Autodesk Inventor part; units mm, degrees
ref_plane "YZ Plane" through (0, 0, 0) normal (1, 0, 0) x (0, 1, 0)
ref_plane "XZ Plane" through (0, 0, 0) normal (0, 1, 0) x (-1, 0, 0)
ref_plane "XY Plane" through (0, 0, 0) normal (0, 0, 1) x (1, 0, 0)
sketch "Skizze1" plane through (0, 0, 0) normal (0, 0, 1) x (1, 0, 0)
  line L0 (0, 0) -> (662.5, 0)
  line L1 (662.5, 0) -> (662.5, 822.5)
  line L2 (662.5, 822.5) -> (0, 822.5)
  line L3 (0, 822.5) -> (0, 0)
  line L4 (0, 822.5) -> (40, 822.5)
  line L5 (40, 822.5) -> (40, 814.5)
  line L6 (40, 814.5) -> (0, 814.5)
  line L7 (0, 814.5) -> (0, 822.5)
  line L8 (0, 822.5) -> (8, 822.5)
  line L9 (8, 822.5) -> (8, 782.5)
  line L10 (8, 782.5) -> (0, 782.5)
  line L11 (0, 782.5) -> (0, 822.5)
  line L12 (0, 411.25) -> (662.5, 411.25) construction
  line L13 (331.25, 822.5) -> (331.25, 0) construction
  line L14 (0, 0) -> (40, 0)
  line L15 (40, 0) -> (40, 8)
  line L16 (40, 8) -> (0, 8)
  line L17 (0, 8) -> (0, 0)
  line L18 (0, 0) -> (8, 0)
  line L19 (8, 0) -> (8, 40)
  line L20 (8, 40) -> (0, 40)
  line L21 (0, 40) -> (0, 0)
  line L22 (662.5, 822.5) -> (662.5, 0)
  line L23 (662.5, 822.5) -> (622.5, 822.5)
  line L24 (622.5, 822.5) -> (622.5, 814.5)
  line L25 (622.5, 814.5) -> (662.5, 814.5)
  line L26 (662.5, 814.5) -> (662.5, 822.5)
  line L27 (662.5, 822.5) -> (654.5, 822.5)
  line L28 (654.5, 822.5) -> (654.5, 782.5)
  line L29 (654.5, 782.5) -> (662.5, 782.5)
  line L30 (662.5, 782.5) -> (662.5, 822.5)
  line L31 (662.5, 0) -> (654.5, 0)
  line L32 (662.5, 0) -> (622.5, 0)
  line L33 (622.5, 0) -> (622.5, 8)
  line L34 (622.5, 8) -> (662.5, 8)
  line L35 (654.5, 0) -> (654.5, 40)
  line L36 (662.5, 8) -> (662.5, 0)
  line L37 (654.5, 40) -> (662.5, 40)
  line L38 (662.5, 40) -> (662.5, 0)
  point P0 (662.5, 782.5)
  point P1 (654.5, 814.5)
  point P2 (8, 814.5)
  point P3 (0, 782.5)
  point P4 (0, 40)
  point P5 (8, 8)
  point P6 (654.5, 8)
  point P7 (662.5, 40)
  dimension "d0" = 662.5
  dimension "d1" = 822.5
  dimension "d2" = 40
  dimension "d3" = 8
  dimension "d4" = 8
  dimension "d5" = 40
extrude "Extrusion1" add sketch "Skizze1" along normal blind 4 contours L15 L16 L19 L20 L3 L10 L9 L6 L5 L2 L24 L25 L28 L29 L1 L37 L35 L34 L33 L0
sketch "Skizze2" plane through (0, 0, 0) normal (0, 0, -1) x (-1, 0, 0)
  line L0 (-624.5, 683.3) -> (-389.5, 683.3)
  line L1 (-389.5, 683.3) -> (-389.5, 284.3)
  line L2 (-389.5, 284.3) -> (-624.5, 284.3)
  line L3 (-624.5, 284.3) -> (-624.5, 683.3)
  line L4 (-654.5, 782.5) -> (-654.5, 814.5)
  line L5 (-654.5, 814.5) -> (-622.5, 814.5)
  point P0 (0, 0)
  dimension "d11" = 399
  dimension "d12" = 235
  dimension "d13" = 30
  dimension "d14" = 131.2
extrude "Extrusion2" cut sketch "Skizze2" against normal up to surface (4 mm away)
sketch "Skizze3" plane through (0, 0, 0) normal (0, 0, -1) x (-1, 0, 0)
  line L0 (0, 782.5) -> (0, 40)
  line L1 (-28, 814.5) -> (0, 814.5)
  line L2 (0, 814.5) -> (0, 694.5)
  line L3 (0, 694.5) -> (-23, 694.5)
  line L4 (-28, 699.5) -> (-28, 814.5)
  line L5 (0, 263) -> (-23, 263)
  line L6 (-28, 258) -> (-28, 143)
  line L7 (-23, 138) -> (0, 138)
  line L8 (0, 138) -> (0, 263)
  line L9 (-8, 40) -> (-8, 8)
  line L10 (-8, 8) -> (-40, 8)
  line L11 (-8, 814.5) -> (-8, 782.5)
  line L12 (-40, 814.5) -> (-8, 814.5)
  arc A0 (-28, 699.5) -> (-23, 694.5) centre (-23, 699.5) ccw
  arc A1 (-23, 263) -> (-28, 258) centre (-23, 258) ccw
  arc A2 (-28, 143) -> (-23, 138) centre (-23, 143) ccw
  point P0 (0, 0)
  point P1 (-28, 694.5)
  point P2 (-28, 263)
  point P3 (0, 138)
  point P4 (0, 686.15)
  point P5 (-28, 138)
  point P6 (0, 138)
  dimension "d17" = 20
  dimension "d19" = 20
  dimension "d20" = 0
  dimension "d21" = 120
  dimension "d61" = 130
  dimension "d62" = 120
  dimension "d63" = 5
  dimension "d64" = 5
extrude "Extrusion3" cut sketch "Skizze3" against normal up to surface (4 mm away)
sketch "Skizze4" plane through (0, 0, 0) normal (0, 0, -1) x (-1, 0, 0)
  line L0 (-619.5, 194.3) -> (-449.5, 194.3)
  line L1 (-444.5, 189.3) -> (-444.5, 159.3)
  line L2 (-449.5, 154.3) -> (-619.5, 154.3)
  line L3 (-624.5, 159.3) -> (-624.5, 189.3)
  line L4 (-624.5, 284.3) -> (-624.5, 683.3)
  line L5 (-389.5, 284.3) -> (-624.5, 284.3)
  arc A0 (-619.5, 194.3) -> (-624.5, 189.3) centre (-619.5, 189.3) ccw
  arc A1 (-624.5, 159.3) -> (-619.5, 154.3) centre (-619.5, 159.3) ccw
  arc A2 (-449.5, 154.3) -> (-444.5, 159.3) centre (-449.5, 159.3) ccw
  arc A3 (-444.5, 189.3) -> (-449.5, 194.3) centre (-449.5, 189.3) ccw
  point P0 (0, 0)
  dimension "d25" = 90
  dimension "d26" = 40
  dimension "d27" = 180
  dimension "d28" = 5
extrude "Extrusion4" cut sketch "Skizze4" against normal up to surface (4 mm away)
sketch "Skizze5" plane through (0, 0, 0) normal (0, 0, -1) x (-1, 0, 0)
  line L0 (-645.9539, 213.8422) -> (-402.4483, 213.8422)
  line L1 (-402.4483, 213.8422) -> (-402.4483, 126.1802)
  line L2 (-402.4483, 126.1802) -> (-645.9539, 126.1802)
  line L3 (-645.9539, 126.1802) -> (-645.9539, 213.8422)
  point P0 (0, 0)
extrude "Extrusion5" add sketch "Skizze5" against normal blind 4
sketch "Skizze6" plane through (0, 0, 0) normal (0, 0, -1) x (-1, 0, 0)
  line L0 (-625.2, 76.6) -> (-592.2, 76.6)
  line L1 (-592.2, 76.6) -> (-592.2, 23.4)
  line L2 (-592.2, 23.4) -> (-625.2, 23.4)
  line L3 (-625.2, 23.4) -> (-625.2, 76.6)
  circle A0 centre (-608.7, 79.25) radius 1.7
  circle A1 centre (-608.7, 20.75) radius 1.7
  line L4 (-40, 0) -> (-622.5, 0)
  line L5 (-662.5, 40) -> (-662.5, 782.5)
  arc A2 (-567.7, 44.7885) -> (-567.7, 55.2115) centre (-558.7, 50) ccw
  line L6 (-567.7, 55.2115) -> (-567.7, 44.7885)
  circle A3 centre (-508.7, 50) radius 11.8
  circle A4 centre (-518.2, 62) radius 1.75
  circle A5 centre (-499.2, 38) radius 1.75
  line L7 (-654.7, 10) -> (-654.7, 0) construction
  line L8 (-654.5, 8) -> (-654.5, 40)
  point P0 (0, 0)
  point P1 (-592.2, 50)
  point P2 (-625.2, 50)
  point P3 (-608.7, 23.4)
  dimension "d33" = 53.2
  dimension "d34" = 33
  dimension "d35" = 16.5
  dimension "d36" = 0
  dimension "d37" = 58.5
  dimension "d38" = 29.25
  dimension "d39" = 3.4
  dimension "d40" = 50
  dimension "d43" = 20.8
  dimension "d44" = 19.4
  dimension "d45" = 0
  dimension "d46" = 50
  dimension "d47" = 24
  dimension "d48" = 12
  dimension "d49" = 23.6
  dimension "d50" = 19
  dimension "d51" = 9.5
  dimension "d52" = 3.5
  dimension "d53" = 0
  dimension "d54" = 50
  dimension "d55" = 10
  dimension "d56" = 0
  dimension "d57" = 0.2
  dimension "d58" = 46
extrude "Extrusion6" cut sketch "Skizze6" against normal blind 4
equation "\"d35\" = 0.5 * d34"
equation "\"d48\" = 0.5 * d47"
equation "\"d51\" = 0.5 * d50"
equation "\"d54\" = d46"
properties part number "101.003.01_Abdeckung_HMI_links" material "PMMA-Kunststoff"
Read the model definition and answer for the solid it produces. Units are mm, in the model's axes. Coordinates: 2 decimals unless noted, no trailing zeros. Loops run counter-clockwise (first coordinate to the right, second up) from the corner with the lowest first, then second, coordinate; pieces in that order, holes last.
(1) Flat-ended cylindrical pins translate along their axes: pin 1 Ø2 at (y, z) = (819.5, 2.5) entering from +X; pin 2 Ø2 at (x, z) = (643, 2.5) entering from -Y. Find the tip coordinate at first contact, or state that the pin passes through.
Solution:
pin 1: stops at x = 622.5
pin 2: stops at y = 8
(2) The part is cut by section A-A (x = 448.5). Determine the outline of the cut face in (y, z), and give its area (3 significant figures).
Solution:
outline: (0, 0) - (284.3, 0) - (284.3, 4) - (0, 4) - close; (683.3, 0) - (822.5, 0) - (822.5, 4) - (683.3, 4) - close
area: 1,690 mm2
(3) The part is cut by section B-B (y = 598). Determine the outline of the cut face in (x, z), and give its area (3 significant figures).
Solution:
outline: (0, 0) - (389.5, 0) - (389.5, 4) - (0, 4) - close; (624.5, 0) - (662.5, 0) - (662.5, 4) - (624.5, 4) - close
area: 1,710 mm2
(4) The part is cut by section C-C (z = 1.1). Count the separate pieces of the cut face and the enclosed holes in it, and give its area (3 significant figures).
Solution:
separate pieces: 1
enclosed holes: 8
area: 440,000 mm2
(5) The mould has two halves that part along X. Classify faces 1 (the face through (253, 417, 0)), 2 (the face through (548.307, 49.619, 1.972)): released by +X, released by -X, zero draft, split by the parting line, or undercut.
Solution:
face 1: zero draft
face 2: undercut
(6) Consider line 1 along X through (y, z) = (296, 2.7); line 2 along Y through (x, z) = (608.7, 2.1); line 3 along X through (y, z) = (79.25, 1.8). Determine where each line is inside the solid, lowest interval first.
Solution:
line 1: x = 0 to 389.5, 624.5 to 662.5
line 2: y = 0 to 19.05, 22.45 to 23.4, 76.6 to 77.55, 80.95 to 284.3, 683.3 to 822.5
line 3: x = 0 to 607, 610.4 to 662.5
